For this review, use the dimensioned drawing (mm, ordinates from the lowest corner) and the shaded views. A direction names the side the tool comes from. Give positions to 0.01 mm unless a question says otherwise; leave off trailing zeros. Order: outer loops, then holes, each group sorted by start corner. A loop starts at its lowest first (then second) coordinate and runs counter-clockwise, first axis right, second up.
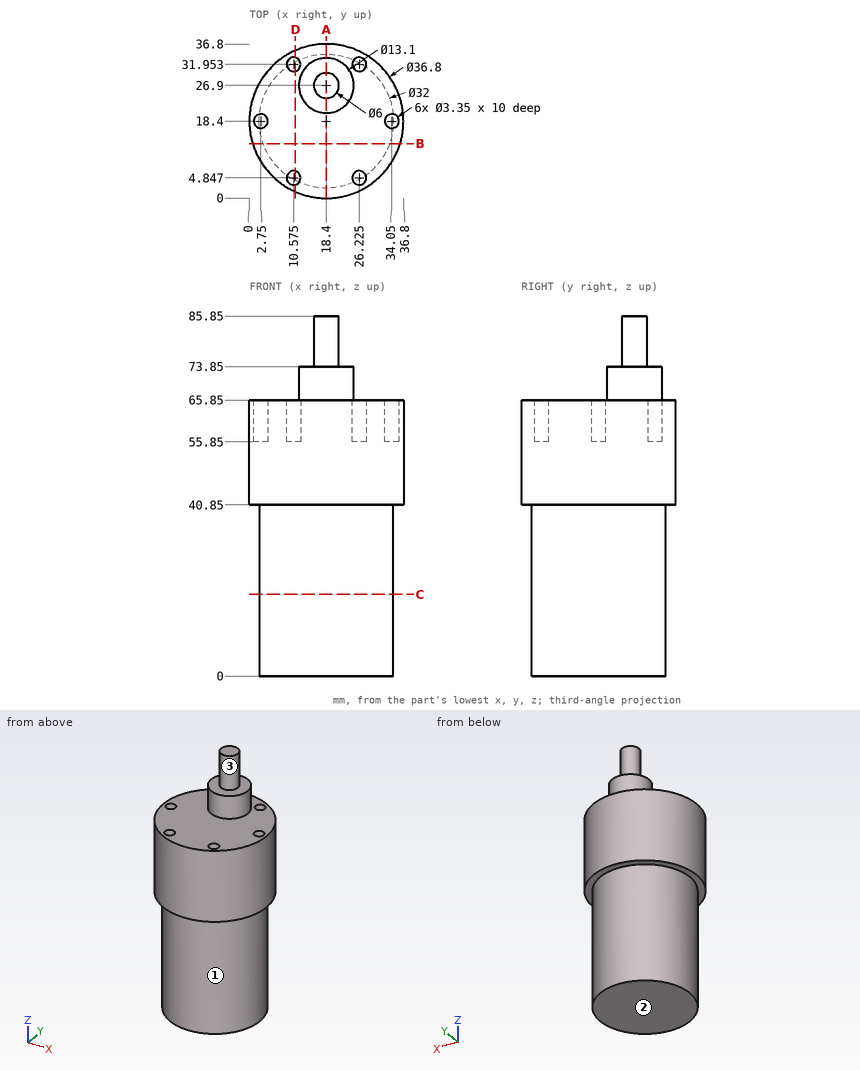
1. For line 1 along Z through (x, y) = (24, 23); line 2 along Z through (x, y) = (14, 34); line 3 along Y through (x, z) = (2, 58) (1 decimal), list the stretches that pass through material, from the lowest coordinate up.
Recorded:
line 1: z = 0 to 65.85
line 2: z = 40.85 to 65.85
line 3: y = 10.1 to 16.9, 19.9 to 26.7
2. Take a section at D-D (x = 11). State the section outline as (y, z) points, then the cut area to 3 significant figures.
Recorded:
outline: (1.55, 40.85) - (4.21, 40.85) - (4.21, 0) - (32.59, 0) - (32.59, 40.85) - (35.25, 40.85) - (35.25, 65.85) - (33.57, 65.85) - (33.57, 55.85) - (30.33, 55.85) - (30.33, 65.85) - (6.47, 65.85) - (6.47, 55.85) - (3.23, 55.85) - (3.23, 65.85) - (1.55, 65.85) - close
area: 1,940 mm2
3. Take a section at A-A (x = 18.4). State the section outline as (y, z) points.
Recorded:
outline: (0, 40.85) - (2.4, 40.85) - (2.4, 0) - (34.4, 0) - (34.4, 40.85) - (36.8, 40.85) - (36.8, 65.85) - (33.45, 65.85) - (33.45, 73.85) - (29.9, 73.85) - (29.9, 85.85) - (23.9, 85.85) - (23.9, 73.85) - (20.35, 73.85) - (20.35, 65.85) - (0, 65.85) - close
4. Machinability: for the marked faces 1, 2 and 3, which of the approach directions +Z, -Z, +X, -X, +Y, -Y give a long, thin tool a straight path to every point of the face, cutting with its end or side? Answer none if there is none.
Recorded:
face 1: -Z
face 2: -Z, +X, -X, +Y, -Y
face 3: +Z
5. Take a section at B-B (y = 13). State the section outline as (x, z) points, then the cut area to 3 significant figures.
Recorded:
outline: (0.81, 40.85) - (3.34, 40.85) - (3.34, 0) - (33.46, 0) - (33.46, 40.85) - (35.99, 40.85) - (35.99, 65.85) - (0.81, 65.85) - close
area: 2,110 mm2
6. Take a section at C-C (z = 19.5). State the section outline as (x, y) points, then the cut area to 3 significant figures.
Recorded:
outline: circle Ø32 at (18.4, 18.4)
area: 804 mm2
7. For pin 1 (2.5 mm diameter, centred on x = 26.22, y = 31.95, fed in from +Z); pin 2 (6 mm diameter, centred on y = 11, z = 55.5, fed in from +X); pin 3 (3 mm diameter, centred on x = 10, y = 9, fed in from +Z); pin 4 (4.5 mm diameter, centred on x = 2.75, y = 18.4, fed in from -Z), all flat-tipped, find the tip position at first contact; note any pin that passes through.
Recorded:
pin 1: stops at z = 55.85
pin 2: stops at x = 36.27
pin 3: stops at z = 65.85
pin 4: stops at z = 0
